from build123d import *

# Parameters (mm, degrees)
SKETCH12_R                = 2.6035
F_10_1010_PROFILE_1_DEPTH = 50.8


with BuildPart() as part:
    # Sketch12 → 10 1010 PROFILE(1) (new body)
    with BuildSketch(Plane(origin=(0, 0, 0), x_dir=(-1, 0, 0), z_dir=(0, 1, 0))):
        with BuildLine():
            Line((-1.709253557, -4.4958), (1.709253557, -4.4958))
            ThreePointArc((1.709253557, -4.4958), (2.922935876, -4.736928798), (3.95226937, -5.423689619))
            Line((3.95226937, -5.423689619), (7.179652728, -8.645192207))
            ThreePointArc((7.179652728, -8.645192207), (7.414733441, -9.822812921), (6.41641086, -10.4902))
            Line((6.41641086, -10.4902), (4.28752, -10.4902))
            ThreePointArc((4.28752, -10.4902), (3.545750844, -10.797450844), (3.2385, -11.53922))
            Line((3.2385, -11.53922), (3.2385, -11.65098))
            ThreePointArc((3.2385, -11.65098), (3.545750844, -12.392749156), (4.28752, -12.7))
            Line((4.28752, -12.7), (5.3171344, -12.7))
            ThreePointArc((5.3171344, -12.7), (5.8251344, -12.192), (6.3331344, -12.7))
            Line((6.3331344, -12.7), (9.5504, -12.7))
            ThreePointArc((9.5504, -12.7), (10.058323491, -12.192000006), (10.566399977, -12.699846982))
            ThreePointArc((10.566399977, -12.699846982), (12.082522516, -12.082522516), (12.699846982, -10.566399977))
            ThreePointArc((12.699846982, -10.566399977), (12.192000006, -10.058323491), (12.7, -9.5504))
            Line((12.7, -9.5504), (12.7, -6.3330836))
            ThreePointArc((12.7, -6.3330836), (12.192, -5.8250836), (12.7, -5.3170836))
            Line((12.7, -5.3170836), (12.7, -4.287470133))
            ThreePointArc((12.7, -4.287470133), (12.392749156, -3.545700977), (11.65098, -3.238450133))
            Line((11.65098, -3.238450133), (11.53922, -3.238450133))
            ThreePointArc((11.53922, -3.238450133), (10.797450844, -3.545700977), (10.4902, -4.287470133))
            Line((10.4902, -4.287470133), (10.4902, -6.402089023))
            ThreePointArc((10.4902, -6.402089023), (9.856394933, -7.351113629), (8.736962546, -7.129240479))
            Line((8.736962546, -7.129240479), (5.440484187, -3.838768792))
            ThreePointArc((5.440484187, -3.838768792), (4.75073678, -2.808015636), (4.5085, -1.591658411))
            Line((4.5085, -1.591658411), (4.5085, 1.591658411))
            ThreePointArc((4.5085, 1.591658411), (4.75073678, 2.808015636), (5.440484187, 3.838768792))
            Line((5.440484187, 3.838768792), (8.736962546, 7.129240479))
            ThreePointArc((8.736962546, 7.129240479), (9.856394933, 7.351113629), (10.4902, 6.402089023))
            Line((10.4902, 6.402089023), (10.4902, 4.287470133))
            ThreePointArc((10.4902, 4.287470133), (10.797450844, 3.545700977), (11.53922, 3.238450133))
            Line((11.53922, 3.238450133), (11.65098, 3.238450133))
            ThreePointArc((11.65098, 3.238450133), (12.392749156, 3.545700977), (12.7, 4.287470133))
            Line((12.7, 4.287470133), (12.7, 5.3171344))
            ThreePointArc((12.7, 5.3171344), (12.192, 5.8251344), (12.7, 6.3331344))
            Line((12.7, 6.3331344), (12.7, 9.5504))
            ThreePointArc((12.7, 9.5504), (12.192000006, 10.058323491), (12.699846982, 10.566399977))
            ThreePointArc((12.699846982, 10.566399977), (12.082522516, 12.082522516), (10.566399977, 12.699846982))
            ThreePointArc((10.566399977, 12.699846982), (10.058323491, 12.192000006), (9.5504, 12.7))
            Line((9.5504, 12.7), (6.3330836, 12.7))
            ThreePointArc((6.3330836, 12.7), (5.8250836, 12.192), (5.3170836, 12.7))
            Line((5.3170836, 12.7), (4.2874692, 12.7))
            ThreePointArc((4.2874692, 12.7), (3.545700044, 12.392749156), (3.2384492, 11.65098))
            Line((3.2384492, 11.65098), (3.2384492, 11.53922))
            ThreePointArc((3.2384492, 11.53922), (3.545700044, 10.797450844), (4.2874692, 10.4902))
            Line((4.2874692, 10.4902), (6.476774195, 10.4902))
            ThreePointArc((6.476774195, 10.4902), (7.43216212, 9.851515102), (7.207191475, 8.724540082))
            Line((7.207191475, 8.724540082), (3.900315394, 5.423689619))
            ThreePointArc((3.900315394, 5.423689619), (2.8709819, 4.736928798), (1.657299581, 4.4958))
            Line((1.657299581, 4.4958), (-1.657299581, 4.4958))
            ThreePointArc((-1.657299581, 4.4958), (-2.8709819, 4.736928798), (-3.900315394, 5.423689619))
            Line((-3.900315394, 5.423689619), (-7.207191475, 8.724540082))
            ThreePointArc((-7.207191475, 8.724540082), (-7.43216212, 9.851515102), (-6.476774195, 10.4902))
            Line((-6.476774195, 10.4902), (-4.2874692, 10.4902))
            ThreePointArc((-4.2874692, 10.4902), (-3.545700044, 10.797450844), (-3.2384492, 11.53922))
            Line((-3.2384492, 11.53922), (-3.2384492, 11.65098))
            ThreePointArc((-3.2384492, 11.65098), (-3.545700044, 12.392749156), (-4.2874692, 12.7))
            Line((-4.2874692, 12.7), (-5.3170836, 12.7))
            ThreePointArc((-5.3170836, 12.7), (-5.8250836, 12.192), (-6.3330836, 12.7))
            Line((-6.3330836, 12.7), (-9.5504, 12.7))
            ThreePointArc((-9.5504, 12.7), (-10.058323491, 12.192000006), (-10.566399977, 12.699846982))
            ThreePointArc((-10.566399977, 12.699846982), (-12.082522516, 12.082522516), (-12.699846982, 10.566399977))
            ThreePointArc((-12.699846982, 10.566399977), (-12.192000006, 10.058323491), (-12.7, 9.5504))
            Line((-12.7, 9.5504), (-12.7, 6.3331344))
            ThreePointArc((-12.7, 6.3331344), (-12.192, 5.8251344), (-12.7, 5.3171344))
            Line((-12.7, 5.3171344), (-12.7, 4.287470133))
            ThreePointArc((-12.7, 4.287470133), (-12.392749156, 3.545700977), (-11.65098, 3.238450133))
            Line((-11.65098, 3.238450133), (-11.53922, 3.238450133))
            ThreePointArc((-11.53922, 3.238450133), (-10.797450844, 3.545700977), (-10.4902, 4.287470133))
            Line((-10.4902, 4.287470133), (-10.4902, 6.402089023))
            ThreePointArc((-10.4902, 6.402089023), (-9.856394933, 7.351113629), (-8.736962546, 7.129240479))
            Line((-8.736962546, 7.129240479), (-5.440484187, 3.838768792))
            ThreePointArc((-5.440484187, 3.838768792), (-4.75073678, 2.808015636), (-4.5085, 1.591658411))
            Line((-4.5085, 1.591658411), (-4.5085, -1.591658411))
            ThreePointArc((-4.5085, -1.591658411), (-4.75073678, -2.808015636), (-5.440484187, -3.838768792))
            Line((-5.440484187, -3.838768792), (-8.736962546, -7.129240479))
            ThreePointArc((-8.736962546, -7.129240479), (-9.856394933, -7.351113629), (-10.4902, -6.402089023))
            Line((-10.4902, -6.402089023), (-10.4902, -4.287470133))
            ThreePointArc((-10.4902, -4.287470133), (-10.797450844, -3.545700977), (-11.53922, -3.238450133))
            Line((-11.53922, -3.238450133), (-11.65098, -3.238450133))
            ThreePointArc((-11.65098, -3.238450133), (-12.392749156, -3.545700977), (-12.7, -4.287470133))
            Line((-12.7, -4.287470133), (-12.7, -5.3170836))
            ThreePointArc((-12.7, -5.3170836), (-12.192, -5.8250836), (-12.7, -6.3330836))
            Line((-12.7, -6.3330836), (-12.7, -9.5504))
            ThreePointArc((-12.7, -9.5504), (-12.192000006, -10.058323491), (-12.699846982, -10.566399977))
            ThreePointArc((-12.699846982, -10.566399977), (-12.082522516, -12.082522516), (-10.566399977, -12.699846982))
            ThreePointArc((-10.566399977, -12.699846982), (-10.058323491, -12.192000006), (-9.5504, -12.7))
            Line((-9.5504, -12.7), (-6.3331344, -12.7))
            ThreePointArc((-6.3331344, -12.7), (-5.8251344, -12.192), (-5.3171344, -12.7))
            Line((-5.3171344, -12.7), (-4.28752, -12.7))
            ThreePointArc((-4.28752, -12.7), (-3.545750844, -12.392749156), (-3.2385, -11.65098))
            Line((-3.2385, -11.65098), (-3.2385, -11.53922))
            ThreePointArc((-3.2385, -11.53922), (-3.545750844, -10.797450844), (-4.28752, -10.4902))
            Line((-4.28752, -10.4902), (-6.41641086, -10.4902))
            ThreePointArc((-6.41641086, -10.4902), (-7.414733441, -9.822812921), (-7.179652728, -8.645192207))
            Line((-7.179652728, -8.645192207), (-3.95226937, -5.423689619))
            ThreePointArc((-3.95226937, -5.423689619), (-2.922935876, -4.736928798), (-1.709253557, -4.4958))
        make_face()
        Circle(SKETCH12_R, mode=Mode.SUBTRACT)
    extrude(amount=F_10_1010_PROFILE_1_DEPTH)


solid = part.part
Input: part model. Units: mm. Frame: model coordinates. A direction names the side the tool comes from. Coordinates: 2 decimals unless noted, no trailing zeros. Loops run counter-clockwise (first coordinate to the right, second up) from the corner with the lowest first, then second, coordinate; pieces in that order, holes last. Notation, with made-up numbers: (74.25, 40) - (116.25, 40) arc R16 cw to (116.25, 61) - close; hole circle Ø8 at (4.25, 62.25). An arc over 180 degrees is marked (long way). Answer in a Markdown table with one row per item. Add a question column.
Item 1: Contact query for flat-ended pins moving along their axis: P1, Ø1.6, axis at y = 34, z = -0.5, coming from the +X side; P2, Ø3, axis at x = 0, z = 0, coming from the -Y side; P3, Ø1.5, axis at y = 35.5, z = -3, coming from the -X side; P4, Ø2.5, axis at x = 0, y = 17.5, coming from the -Z side. Output: stop coordinate, or through.
Item 2: Mould query, pull axis Z, two halves, no side actions, for faces 1 (the cylindrical face through (12.192, 25.044, -10.047)), 2 (the cylindrical face through (-10.047, 25.044, -12.192)), 3 (the flat face through (-12.7, 25, 8)). Classes: released by +Z, released by -Z, zero draft, split by the parting line, or undercut.
Item 3: Section query A-A on z = 0. Return the cut outline in (x, y), then the cut area to 3 significant figures.
Item 4: Section query B-B on x = 0. Return the cut outline in (y, z).
Item 5: Line query: line 1 along Z through (x, y) = (0, 16); line 2 along X through (y, z) = (47.5, -5.75); line 3 along X through (y, z) = (40, 3.75). Output: solid intervals per line, ascending. Write a range as [from, to].
Item 6: Access query for faces 4 (the cylindrical face through (3.538, 25.044, 12.385)), 5 (the cylindrical face through (3.554, 25.044, -12.401)), 6 (the flat face through (-4.508, 25, 0)), 7 (the cylindrical face through (-10.789, 25.044, 3.554)). Directions: +Z, -Z, +X, -X, +Y, -Y. A direction counts if a zero-diameter tool reaches every point of the face in a straight line with its end or side. Return the directions, or none.
Recorded:
| question | item | result |
|---|---|---|
| 1 | P1 | x = 4.51 |
| 1 | P2 | through |
| 1 | P3 | x = -12.55 |
| 1 | P4 | z = -4.5 |
| 2 | face 1 | undercut |
| 2 | face 2 | released by -Z |
| 2 | face 3 | zero draft |
| 3 | outline | (-4.51, 0) - (-2.6, 0) - (-2.6, 50.8) - (-4.51, 50.8) - close; (2.6, 0) - (4.51, 0) - (4.51, 50.8) - (2.6, 50.8) - close |
| 3 | area | 194 mm^2 |
| 4 | outline | (0, -4.5) - (50.8, -4.5) - (50.8, -2.6) - (0, -2.6) - close; (0, 2.6) - (50.8, 2.6) - (50.8, 4.5) - (0, 4.5) - close |
| 5 | line 1 | [-4.5, -2.6], [2.6, 4.5] |
| 5 | line 2 | [-12.2, -10.49], [-7.36, -4.28], [4.28, 7.36], [10.49, 12.2] |
| 5 | line 3 | [-12.55, -10.64], [-5.35, 5.35], [10.64, 12.55] |
| 6 | face 4 | +Z, +Y, -Y |
| 6 | face 5 | -Z, +Y, -Y |
| 6 | face 6 | -X, +Y, -Y |
| 6 | face 7 | +Y, -Y |
